Input: part model. Units: mm. Frame: model coordinates. A direction names the side the tool comes from. Coordinates: 2 decimals unless noted, no trailing zeros. Write each loop counter-clockwise with the first axis right and the second up, starting at its lowest first coordinate (ties: lowest second). Pieces come first, ordered by that corner, then holes. Notation, with made-up numbers: M 72.5,67 L 119.5,67 A5 ccw 119.5,73 Z; hole C -39,-5 d9. An arc over 180 degrees is marked long. Use one line per item in the form item = value.
from build123d import *

# Parameters (mm, degrees)
F0_W     = 15
F0_H     = 10
F0_W_2   = 10
F0_H_2   = 15
F0_H_3   = 12
F0_W_3   = 12
F1_DEPTH = 100
F2_R     = 5


with BuildPart() as f1:
    # F0 (on Front) → F1 (new body)
    with BuildSketch(Plane.XZ):
        Polygon((10.2, -7.5), (10.2, -15.2), (7.5, -15.2), (7.5, -25.2), (20.2, -25.2), (20.2, -7.5), align=None)
        with Locations((0, -20.2)):
            Rectangle(F0_W, F0_H)
        with Locations((15.2, 0)):
            Rectangle(F0_W_2, F0_H_2)
        Polygon((-7.5, -25.2), (-7.5, -15.2), (-10.2, -15.2), (-10.2, -7.5), (-20.2, -7.5), (-20.2, -25.2), align=None)
        with Locations((0, -31.2)):
            Rectangle(F0_W, F0_H_3)
        Polygon((10.2, 15.2), (10.2, 7.5), (20.2, 7.5), (20.2, 25.2), (7.5, 25.2), (7.5, 15.2), align=None)
        with Locations((26.2, 0)):
            Rectangle(F0_W_3, F0_H_2)
        with Locations((-15.2, 0)):
            Rectangle(F0_W_2, F0_H_2)
        with Locations((0, 20.2)):
            Rectangle(F0_W, F0_H)
        Polygon((-20.2, 7.5), (-10.2, 7.5), (-10.2, 15.2), (-7.5, 15.2), (-7.5, 25.2), (-20.2, 25.2), align=None)
        with Locations((-26.2, 0)):
            Rectangle(F0_W_3, F0_H_2)
        with Locations((0, 31.2)):
            Rectangle(F0_W, F0_H_3)
    extrude(amount=F1_DEPTH)

    # F2
    f2_edges = [f1.edges().sort_by_distance(p)[0] for p in [
        (-20.2, -50, 25.2),
        (20.2, -50, 25.2),
        (20.2, -50, -25.2),
        (-20.2, -50, -25.2),
        (32.2, -50, 7.5),
        (32.2, -50, -7.5),
        (20.2, -50, 7.5),
        (20.2, -50, -7.5),
        (7.5, -50, 25.2),
        (7.5, -50, 37.2),
        (-7.5, -50, 37.2),
        (-7.5, -50, 25.2),
        (-20.2, -50, 7.5),
        (-32.2, -50, 7.5),
        (-32.2, -50, -7.5),
        (-32.2, 0, 0),
        (-32.2, -100, 0),
        (-20.2, -50, -7.5),
        (-7.5, -50, -25.2),
        (-7.5, -50, -37.2),
        (7.5, -50, -37.2),
        (0, 0, -37.2),
        (0, -100, -37.2),
        (7.5, -50, -25.2),
    ]]
    fillet(f2_edges, radius=F2_R)


solid = f1.part
(1) First-contact query: pin 1 Ø4 at (y, z) = (-49, -16.5) entering from +X; pin 2 Ø1.3 at (x, y) = (-14, -56) entering from +Z; pin 3 Ø3 at (x, y) = (14, -63) entering from -Z; pin 4 Ø12 at (x, z) = (3, -6.5) entering from +Y. Flat tips, straight axial feed; report the tip coordinate or a pass-through.
Computed:
pin_1 = 20.2
pin_2 = 25.2
pin_3 = -25.2
pin_4 = through
(2) Set-up query: faces 4 (the flat face through (20.2, -49, -16)), 5 (the cylindrical face through (-18.7, -50.7, 23.77)), 6 (the flat face through (14, -49, 25.2)). Return all of +Z, -Z, +X, -X, +Y, -Y with unobstructed straight access to the full face (end or side cutting, diameter ignored); none if empty.
Computed:
face_4 = -Z, +X, +Y, -Y
face_5 = +Z, -X, +Y, -Y
face_6 = +Z, +X, +Y, -Y
(3) Section query C-C on x = -23. Return the cut outline in (y, z), plus the area to 3 significant figures.
Computed:
outline = M -100,-8.01 L 0,-8.01 L 0,8.01 L -100,8.01 Z
area = 1,600 mm^2
(4) Section query A-A on x = -4.5. Return the cut outline in (y, z), plus the area to 3 significant figures.
Computed:
outline = M -100,-32.2 A5 ccw -97,-36.78 L -3,-36.78 A5 ccw 0,-32.2 L 0,-15.2 L -100,-15.2 Z; M -100,15.2 L 0,15.2 L 0,36.78 L -100,36.78 Z
area = 4,310 mm^2
(5) Section query B-B on z = 11. Return the cut outline in (x, y).
Computed:
outline = M -20.43,-100 L -10.2,-100 L -10.2,0 L -20.43,0 Z; M 10.2,-100 L 20.43,-100 L 20.43,0 L 10.2,0 Z
(6) Pull-direction query (Z, two-part tool) for faces 1 (the flat face through (10.2, -49, 0)), 2 (the cylindrical face through (21.63, -50.7, -9)), 3 (the cylindrical face through (30.77, -50.7, 6)); classes: pulls with the +Z half, pulls with the -Z half, needs draft (parallel to the pull), parting line crosses it, or undercut.
Computed:
face_1 = undercut
face_2 = pulls with the -Z half
face_3 = pulls with the +Z half
(7) Line query: probe 1 along X at (y, z) = (-31, 2); probe 2 along X at (y, z) = (-32, -15); probe 3 along Z at (x, y) = (8.5, -49). Output: solid intervals per line, ascending.
Computed:
probe_1 = -32.2 to -10.2, 10.2 to 32.2
probe_2 = -20.2 to -10.2, 10.2 to 20.2
probe_3 = -27.2 to -15.2, 15.2 to 27.2
